```python
from build123d import *

# Parameters (mm, degrees)
BOSS_EXTRUDE1_DEPTH      = 6
BOSS_EXTRUDE2_DEPTH      = 40
CUT_EXTRUDE1_REACH       = 62.762
SKETCH9_R                = 1.5
CUT_EXTRUDE2_REACH       = 62.762
SKETCH10_R               = 7.5
BOSS_EXTRUDE4_DEPTH      = 25
BOSS_EXTRUDE5_REACH      = 73.576
BOSS_EXTRUDE5_END_RADIUS = 23.4
SKETCH12_R               = 2.5
BOSS_EXTRUDE6_REACH      = 73.576
SKETCH14_R               = 2.5


with BuildPart() as part:
    # Sketch3 → Boss-Extrude1 (new body)
    with BuildSketch(Plane.XY):
        with BuildLine():
            Line((-20, 10.240601504), (20, 10.240601504))
            ThreePointArc((20, 10.240601504), (24.242640687, 8.483242191), (26, 4.240601504))
            Line((26, 4.240601504), (26, -13.759398496))
            ThreePointArc((26, -13.759398496), (24.242640687, -18.002039183), (20, -19.759398496))
            Line((20, -19.759398496), (-20, -19.759398496))
            ThreePointArc((-20, -19.759398496), (-24.242640687, -18.002039183), (-26, -13.759398496))
            Line((-26, -13.759398496), (-26, 4.240601504))
            ThreePointArc((-26, 4.240601504), (-24.242640687, 8.483242191), (-20, 10.240601504))
        make_face()
    extrude(amount=BOSS_EXTRUDE1_DEPTH)

    # Sketch4 → Boss-Extrude2 (add)
    with BuildSketch(Plane.XY.offset(6)):
        with BuildLine():
            Line((-26, 4.240601504), (26, 4.240601504))
            ThreePointArc((26, 4.240601504), (24.242640687, 8.483242191), (20, 10.240601504))
            Line((20, 10.240601504), (-20, 10.240601504))
            ThreePointArc((-20, 10.240601504), (-24.242640687, 8.483242191), (-26, 4.240601504))
        make_face()
    extrude(amount=BOSS_EXTRUDE2_DEPTH)

    # Sketch9 → Cut-Extrude1 (cut, up to next)
    with BuildSketch(Plane(origin=(0, 10.240601504, 0), x_dir=(1, 0, 0), z_dir=(0, 1, 0)), mode=Mode.PRIVATE) as cut_extrude1_sk1:
        with Locations(Location((0, -41.5, 0), (0, 0, 180))):
            Circle(SKETCH9_R)
    cut_extrude1_tool1 = extrude(cut_extrude1_sk1.sketch, amount=-CUT_EXTRUDE1_REACH, mode=Mode.PRIVATE) & part.part
    # Sketch9 → Cut-Extrude1 (cut, up to next)
    with BuildSketch(Plane(origin=(0, 10.240601504, 0), x_dir=(1, 0, 0), z_dir=(0, 1, 0)), mode=Mode.PRIVATE) as cut_extrude1_sk2:
        with Locations(Location((13.423393759, -33.75, 0), (0, 0, 180))):
            Circle(SKETCH9_R)
    cut_extrude1_tool2 = extrude(cut_extrude1_sk2.sketch, amount=-CUT_EXTRUDE1_REACH, mode=Mode.PRIVATE) & part.part
    # Sketch9 → Cut-Extrude1 (cut, up to next)
    with BuildSketch(Plane(origin=(0, 10.240601504, 0), x_dir=(1, 0, 0), z_dir=(0, 1, 0)), mode=Mode.PRIVATE) as cut_extrude1_sk3:
        with Locations(Location((-13.423393759, -33.75, 0), (0, 0, 180))):
            Circle(SKETCH9_R)
    cut_extrude1_tool3 = extrude(cut_extrude1_sk3.sketch, amount=-CUT_EXTRUDE1_REACH, mode=Mode.PRIVATE) & part.part
    # Sketch9 → Cut-Extrude1 (cut, up to next)
    with BuildSketch(Plane(origin=(0, 10.240601504, 0), x_dir=(1, 0, 0), z_dir=(0, 1, 0)), mode=Mode.PRIVATE) as cut_extrude1_sk4:
        with Locations(Location((-13.423393759, -18.25, 0), (0, 0, 180))):
            Circle(SKETCH9_R)
    cut_extrude1_tool4 = extrude(cut_extrude1_sk4.sketch, amount=-CUT_EXTRUDE1_REACH, mode=Mode.PRIVATE) & part.part
    # Sketch9 → Cut-Extrude1 (cut, up to next)
    with BuildSketch(Plane(origin=(0, 10.240601504, 0), x_dir=(1, 0, 0), z_dir=(0, 1, 0)), mode=Mode.PRIVATE) as cut_extrude1_sk5:
        with Locations(Location((0, -10.5, 0), (0, 0, 180))):
            Circle(SKETCH9_R)
    cut_extrude1_tool5 = extrude(cut_extrude1_sk5.sketch, amount=-CUT_EXTRUDE1_REACH, mode=Mode.PRIVATE) & part.part
    # Sketch9 → Cut-Extrude1 (cut, up to next)
    with BuildSketch(Plane(origin=(0, 10.240601504, 0), x_dir=(1, 0, 0), z_dir=(0, 1, 0)), mode=Mode.PRIVATE) as cut_extrude1_sk6:
        with Locations(Location((13.423393759, -18.25, 0), (0, 0, 180))):
            Circle(SKETCH9_R)
    cut_extrude1_tool6 = extrude(cut_extrude1_sk6.sketch, amount=-CUT_EXTRUDE1_REACH, mode=Mode.PRIVATE) & part.part
    add(cut_extrude1_tool1.solids().sort_by_distance((0, 10.240602, 41.5))[0], mode=Mode.SUBTRACT)
    add(cut_extrude1_tool2.solids().sort_by_distance((13.423394, 10.240602, 33.75))[0], mode=Mode.SUBTRACT)
    add(cut_extrude1_tool3.solids().sort_by_distance((-13.423394, 10.240602, 33.75))[0], mode=Mode.SUBTRACT)
    add(cut_extrude1_tool4.solids().sort_by_distance((-13.423394, 10.240602, 18.25))[0], mode=Mode.SUBTRACT)
    add(cut_extrude1_tool5.solids().sort_by_distance((0, 10.240602, 10.5))[0], mode=Mode.SUBTRACT)
    add(cut_extrude1_tool6.solids().sort_by_distance((13.423394, 10.240602, 18.25))[0], mode=Mode.SUBTRACT)

    # Sketch10 → Cut-Extrude2 (cut, up to next)
    with BuildSketch(Plane(origin=(0, 10.240601504, 0), x_dir=(1, 0, 0), z_dir=(0, 1, 0)), mode=Mode.PRIVATE) as cut_extrude2_sk1:
        with Locations(Location((-5.5, -26, 0), (0, 0, 180))):
            Circle(SKETCH10_R)
    cut_extrude2_tool1 = extrude(cut_extrude2_sk1.sketch, amount=-CUT_EXTRUDE2_REACH, mode=Mode.PRIVATE) & part.part
    add(cut_extrude2_tool1.solids().sort_by_distance((-5.5, 10.240602, 26))[0], mode=Mode.SUBTRACT)

    # Sketch11 → Boss-Extrude4 (add)
    with BuildSketch(Plane(origin=(0, 10.240601504, 0), x_dir=(1, 0, 0), z_dir=(0, 1, 0))):
        with BuildLine():
            Line((16.755404651, -17.041405524), (20.209569094, -14.204521331))
            ThreePointArc((20.209569094, -14.204521331), (0.448372053, -2.604296067), (-19.742781111, -13.438845833))
            Line((-19.742781111, -13.438845833), (-16.246095761, -16.147874721))
            ThreePointArc((-16.246095761, -16.147874721), (0.514245282, -7.006960438), (16.755404651, -17.041405524))
        make_face()
    extrude(amount=BOSS_EXTRUDE4_DEPTH)

    # Boss-Extrude5: up to this cylinder (the profile starts outside it)
    boss_extrude5_end = Plane(origin=(0, 6.683051, 26), z_dir=(0, -1, 0)) * Cylinder(BOSS_EXTRUDE5_END_RADIUS, 194.952, mode=Mode.PRIVATE)
    # Sketch12 → Boss-Extrude5 (add, up to the surface)
    with BuildSketch(Plane(origin=(7.879699248, -7.879699248, 0), x_dir=(0, 0, 1), z_dir=(-0.7071067811865489, 0.7071067811865462, 0)), mode=Mode.PRIVATE) as boss_extrude5_sk1:
        with Locations((7.574761701, 20.594839086)):
            Circle(SKETCH12_R)
    boss_extrude5_tool1 = extrude(boss_extrude5_sk1.sketch, amount=BOSS_EXTRUDE5_REACH, mode=Mode.PRIVATE) - boss_extrude5_end
    add(boss_extrude5_tool1.solids().sort_by_distance((22.44245, 6.683051, 7.574762))[0])

    # Sketch14 → Boss-Extrude6 (add, up to next)
    with BuildSketch(Plane(origin=(-7.879699248, -7.879699248, 0), x_dir=(0, 0, -1), z_dir=(0.7071067811865487, 0.7071067811865465, 0)), mode=Mode.PRIVATE) as boss_extrude6_sk1:
        with Locations((-10.283332747, 20.780524406)):
            Circle(SKETCH14_R)
    boss_extrude6_tool1 = extrude(boss_extrude6_sk1.sketch, amount=BOSS_EXTRUDE6_REACH, mode=Mode.PRIVATE) - part.part
    add(boss_extrude6_tool1.solids().sort_by_distance((-22.573749, 6.81435, 10.283333))[0])


solid = part.part
```
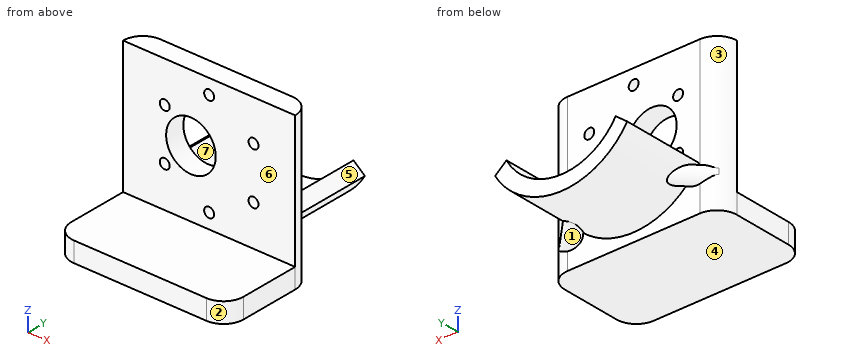
Here's how the part is built. I have some questions about the finished solid (model axes, mm). Face numbers are marked on the shaded views. A direction names the side the tool comes from. Coordinates: 2 decimals unless noted, no trailing zeros. Order: outer loops, then holes, each group sorted by start corner. A loop starts at its lowest first (then second) coordinate and runs counter-clockwise, first axis right, second up. Notation, with made-up numbers: (-20, 76.5) -> (10, 76.5) arc R30 ccw to (10, 104.5) -> close; hole circle Ø1 at (2, 23.5). An arc over 180 degrees is marked (long way). Return JSON: item names as keys, results as strings.
1) On a 3-axis mill with a long thin cutter (end or side, diameter ignored), from which of +Z, -Z, +X, -X, +Y, -Y can I reach the whole of each face in a straight line? I mean the marked faces 4, 5, 6 and 7. Say none if no direction works.
Conclusion:
{"face 4": "-Z, +X, -X, +Y, -Y", "face 5": "+Z, +X, +Y", "face 6": "+Z, +X, -X, -Y", "face 7": "+Z, +Y"}
2) If we section it at B-B on x = -5.5: List the corners of the cut face in (y, z) for me.
Conclusion:
{"outline": "(-19.76, 0) -> (10.24, 0) -> (10.24, 3.26) -> (35.24, 3.26) -> (35.24, 7.81) -> (10.24, 7.81) -> (10.24, 18.5) -> (4.24, 18.5) -> (4.24, 6) -> (-19.76, 6) -> close; (4.24, 33.5) -> (10.24, 33.5) -> (10.24, 46) -> (4.24, 46) -> close"}
3) If we section it at C-C on x = 0: List the corners of the cut face in (y, z) for me, plus the area to 3 significant figures.
Conclusion:
{"outline": "(-19.76, 0) -> (10.24, 0) -> (10.24, 2.6) -> (35.24, 2.6) -> (35.24, 7) -> (10.24, 7) -> (10.24, 9) -> (4.24, 9) -> (4.24, 6) -> (-19.76, 6) -> close; (4.24, 12) -> (10.24, 12) -> (10.24, 20.9) -> (4.24, 20.9) -> close; (4.24, 31.1) -> (10.24, 31.1) -> (10.24, 40) -> (4.24, 40) -> close; (4.24, 43) -> (10.24, 43) -> (10.24, 46) -> (4.24, 46) -> close", "area": "433 mm²"}
4) If I drill on probe 1 along X at (y, z) = (7, 18); probe 2 along Z at (x, y) = (-5.5, 7); probe 3 along Y at (x, z) = (10, 22.5), over which ranges is the centre line in solid material (lowest first)?
Conclusion:
{"probe 1": "x = -25.33 to -14.9, -11.94 to 11.94, 14.9 to 25.33", "probe 2": "z = 0 to 18.5, 33.5 to 46", "probe 3": "y = 4.24 to 10.24"}
5) Thinking about a two-plate mould opening in X: for the marked faces 1, 2 and 3, which applies, +X half, -X half, draft (parallel to the pull), parting line (faces both ways), or undercut?
Conclusion:
{"face 1": "undercut", "face 2": "+X half", "face 3": "-X half"}
6) If we section it at A-A on z = 26: List the corners of the cut face in (x, y) for me.
Conclusion:
{"outline": "(-26, 4.24) -> (-13, 4.24) -> (-13, 10.24) -> (-20, 10.24) arc R6 ccw to start; (2, 4.24) -> (26, 4.24) arc R6 ccw to (20, 10.24) -> (2, 10.24) -> close"}
7) If we section it at D-D on y = -6: List the corners of the cut face in (x, z) for me.
Conclusion:
{"outline": "(-26, 0) -> (26, 0) -> (26, 6) -> (-26, 6) -> close"}
8) I'm going to push flat-ended pins straight in: P1, Ø5, axis at x = 13.42, z = 18.25, coming from the -Y side; P2, Ø2, axis at x = -5, y = 18.5, coming from the +Z side; P3, Ø5, axis at x = 4, y = -1.5, coming from the +Z side. Where does each tip first touch, or does it pass through?
Conclusion:
{"P1": "stops at y = 4.24", "P2": "stops at z = 7.97", "P3": "stops at z = 6"}
